Solid Edge part; units mm, degrees
sketch "Sketch1" plane through (0, 38.5, 0) normal (0, -1, 0) x (1, 0, 0)
  line L0 (-20, -0.4056) -> (10.4056, 30)
  line L1 (10.4056, 30) -> (-20, 60.4056)
  line L2 (-20, 60.4056) -> (-50.4056, 30)
  line L3 (-50.4056, 30) -> (-20, -0.4056)
  dimension "D1" = 20
extrude "ExtrudedProtrusion_1" add sketch "Sketch1" against normal blind 8
sketch "Sketch2" plane through (0, 38.5, 0) normal (0, -1, 0) x (1, 0, 0)
  line L0 (0, 0) -> (0, 19.5944)
  line L1 (0, 19.5944) -> (-10, 9.5944)
  line L2 (-10, 9.5944) -> (-10, 0)
  line L3 (-10, 0) -> (0, 0)
extrude "ExtrudedProtrusion_2" add sketch "Sketch2" against normal blind 60
sketch "Sketch3" plane through (0, 38.5, 0) normal (0, -1, 0) x (1, 0, 0)
  line L0 (0, 19) -> (10.4056, 19)
  line L1 (10.4056, 19) -> (10.4056, 30)
  line L2 (10.4056, 30) -> (0, 19.5944)
  line L3 (0, 19.5944) -> (0, 19)
extrude "ExtrudedProtrusion_3" add sketch "Sketch3" against normal blind 60
hole "Hole_1" at (-20, 46.5, 30) direction (0, -1, 0) diameter 25 end up to next
hole "Hole_2" at (1.9203, 46.5, 30) direction (0, -1, 0) diameter 3.6 end up to next
hole "Hole1" at (-20, 46.5, 51.9203) direction (0, -1, 0) diameter 3.6 end up to next
hole "Hole2" at (-41.9203, 46.5, 30) direction (0, -1, 0) diameter 3.6 end up to next
hole "Hole3" at (-20, 46.5, 8.0797) direction (0, -1, 0) diameter 3.6 end up to next
chamfer "Chamfer_1" distance 3 angle 45 3 edges at (-20, 42.5, 60.4056) (-50.4056, 42.5, 30) (-20, 42.5, -0.4056)
sketch "Sketch4" plane through (-5, 68.5, 0) normal (0, 0, -1) x (0, -1, 0)
  line L0 (-30, 5) -> (-30, -5)
  line L1 (30, -5) -> (-30, -5)
  line L2 (30, 5) -> (30, -5)
  line L3 (-30, 5) -> (30, 5)
extrude "ExtrudedProtrusion_5" add sketch "Sketch4" along normal blind 15
hole "Hole_6" at (-10, 48.5, 0) direction (1, 0, 0) diameter 5 end up to next
hole "Hole4" at (-10, 68.5, 0) direction (1, 0, 0) diameter 5 end up to next
properties material "Polyethylene, low density"
Verification items for the finished model (mm, model axes). A direction names the side the tool comes from. Give positions to 0.01 mm unless a question says otherwise; leave off trailing zeros. Write each loop counter-clockwise with the first axis right and the second up, starting at its lowest first coordinate (ties: lowest second). Pieces come first, ordered by that corner, then holes. Notation, with made-up numbers: (8, 35) - (33, 35) arc R7 cw to (33, 40) - close; hole circle Ø1 at (79.5, 71). An arc over 180 degrees is marked (long way). Put each result on its own line as item: value.
Q1. Mould release check, pull along X, two halves, no side actions. Record for faces 1 (the face through (-48.284, 43, 30)), 2 (the face through (-20, 43, 1.716)), 3 (the face through (2.461, 42.556, 31.717)): released by +X, released by -X, zero draft, split by the parting line, or undercut.
Result:
face 1: released by -X
face 2: zero draft
face 3: undercut
Q2. Section check D-D on z = 34.5. Record the cut outline in (x, y).
Result:
outline: (-45.91, 38.5) - (-31.66, 38.5) - (-31.66, 46.5) - (-45.91, 46.5) - close; (-8.34, 38.5) - (5.91, 38.5) - (5.91, 46.5) - (-8.34, 46.5) - close
Q3. Depth check by flat-ended pin: P1, Ø2, axis at x = -21, y = 41.5, coming from the -Z side; P2, Ø6, axis at x = -30, z = 15, coming from the +Y side; P3, Ø12, axis at x = 2.5, y = 91, coming from the +Z side. Enter the tip coordinate at first touch or a pass-through.
Result:
P1: z = 1.72
P2: y = 46.5
P3: z = 28.09
Q4. Scan lines: probe 1 along Y at (x, z) = (-6.5, 0); probe 2 along Z at (x, y) = (-20, 41.5); probe 3 along X at (y, z) = (40.75, 30). Record each from-to range of solid material in increasing order. Write a range as from..to.
Result:
probe 1: 38.5..46, 51..66, 71..98.5
probe 2: 1.72..6.28, 9.88..17.5, 42.5..50.12, 53.72..58.28
probe 3: -48.28..-43.72, -40.12..-32.5, -7.5..0.12, 3.72..10.41
Q5. Section check C-C on x = -8.5. Record the cut outline in (y, z), and give its area (3 significant figures).
Result:
outline: (38.5, -15) - (98.5, -15) - (98.5, 11.09) - (46.5, 11.09) - (46.5, 25.1) - (38.5, 25.1) - close; (38.5, 34.9) - (46.5, 34.9) - (46.5, 48.91) - (38.5, 48.91) - close; hole circle Ø5 at (48.5, 0); hole circle Ø5 at (68.5, 0)
area: 1,750 mm2
Q6. Section check B-B on y = 70. Record the cut outline in (x, z).
Result:
outline: (-10, -15) - (0, -15) - (0, -2) - (-10, -2) - close; (-10, 2) - (0, 2) - (0, 19) - (10.41, 19) - (10.41, 30) - (-10, 9.59) - close
Q7. Set-up check for faces 4 (the face through (-13.994, 42.444, 5.6)), 5 (the face through (0.346, 72.136, 19.94)), 6 (the face through (0, 68, 6)): record each of +Z, -Z, +X, -X, +Y, -Y from which the full face is reachable in a straight line by a thin tool's end or side.
Result:
face 4: -Z, +Y, -Y
face 5: +Z, -X, +Y
face 6: -Z, +X, +Y, -Y
Q8. Section check A-A on z = 0. Record the cut outline in (x, y).
Result:
outline: (-10, 38.5) - (0, 38.5) - (0, 46) - (-10, 46) - close; (-10, 51) - (0, 51) - (0, 66) - (-10, 66) - close; (-10, 71) - (0, 71) - (0, 98.5) - (-10, 98.5) - close
